from build123d import *

# Parameters (mm, degrees)
SKETCH1_W           = 30
SKETCH1_H           = 10
BOSS_EXTRUDE1_DEPTH = 0.6
SKETCH2_W           = 0.6
SKETCH2_H           = 10
BOSS_EXTRUDE2_DEPTH = 10
FILLET1_R           = 0.5
FILLET2_R           = 3
CUT_EXTRUDE1_REACH  = 2.6
SKETCH3_R           = 2.5


with BuildPart() as part:
    # Sketch1 → Boss-Extrude1 (new body)
    with BuildSketch(Plane(origin=(0, 0, 0), x_dir=(1, 0, 0), z_dir=(0, 1, 0))):
        Rectangle(SKETCH1_W, SKETCH1_H)
    extrude(amount=BOSS_EXTRUDE1_DEPTH)

    # Sketch2 → Boss-Extrude2 (add)
    with BuildSketch(Plane(origin=(0, 0.6, 0), x_dir=(1, 0, 0), z_dir=(0, 1, 0))):
        with Locations((-14.7, 0)):
            Rectangle(SKETCH2_W, SKETCH2_H)
        with Locations((14.7, 0)):
            Rectangle(SKETCH2_W, SKETCH2_H)
    extrude(amount=BOSS_EXTRUDE2_DEPTH)

    # Fillet1
    fillet1_edges = [part.edges().sort_by_distance(p)[0] for p in [
        (-14.4, 0.6, 0),
        (14.4, 0.6, 0),
        (-15, 0, 0),
        (15, 0, 0),
    ]]
    fillet(fillet1_edges, radius=FILLET1_R)

    # Fillet2
    fillet2_edges = [part.edges().sort_by_distance(p)[0] for p in [
        (-14.7, 10.6, 5),
        (-14.7, 10.6, -5),
        (14.7, 10.6, -5),
        (14.7, 10.6, 5),
    ]]
    fillet(fillet2_edges, radius=FILLET2_R)

    # Sketch3 → Cut-Extrude1 (cut, up to next)
    with BuildSketch(Plane(origin=(0, 0.6, 0), x_dir=(1, 0, 0), z_dir=(0, 1, 0)), mode=Mode.PRIVATE) as cut_extrude1_sk1:
        Circle(SKETCH3_R)
    cut_extrude1_tool1 = extrude(cut_extrude1_sk1.sketch, amount=-CUT_EXTRUDE1_REACH, mode=Mode.PRIVATE) & part.part
    add(cut_extrude1_tool1.solids().sort_by_distance((0, 0.6, 0))[0], mode=Mode.SUBTRACT)


solid = part.part
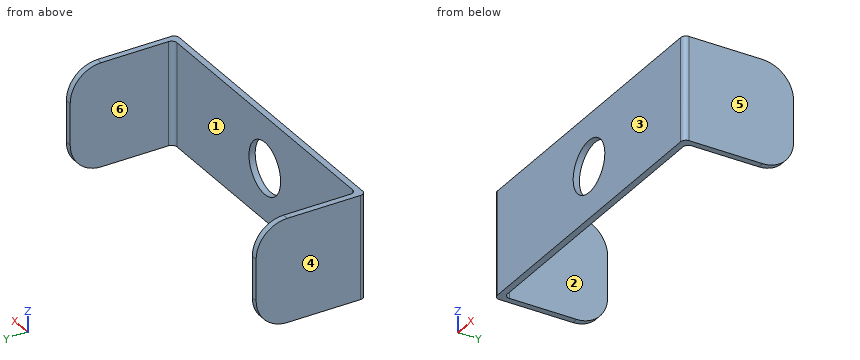
CAD build for the part. Positions are in the model's coordinates, mm. Face numbers are marked on the shaded views. A direction names the side the tool comes from. Give positions to 0.01 mm unless a question says otherwise; leave off trailing zeros. Write each loop counter-clockwise with the first axis right and the second up, starting at its lowest first coordinate (ties: lowest second). Pieces come first, ordered by that corner, then holes. Notation, with made-up numbers: (46.5, -14.5) - (60.5, -14.5) arc R13 cw to (60.5, -10.5) - close; hole circle Ø1 at (14.5, 34). An arc over 180 degrees is marked (long way). Answer as CSV lines item,"result".
Q1. Band-saw the part on B-B (z = 0). Give the cut face in (x, y), and give its area (3 significant figures).
Result set:
outline,"(-15, 0.5) arc R0.5 ccw to (-14.5, 0) - (-2.5, 0) - (-2.5, 0.6) - (-13.9, 0.6) arc R0.5 cw to (-14.4, 1.1) - (-14.4, 10.6) - (-15, 10.6) - close; (2.5, 0) - (14.5, 0) arc R0.5 ccw to (15, 0.5) - (15, 10.6) - (14.4, 10.6) - (14.4, 1.1) arc R0.5 cw to (13.9, 0.6) - (2.5, 0.6) - close"
area,"27.0 mm²"
Q2. Pull direction X, two halves, no side cores. Call the marked faces 1, 2, 3 and 4: released by +X, released by -X, zero draft, split by the parting line, or undercut.
Result set:
face 1,"undercut"
face 2,"undercut"
face 3,"zero draft"
face 4,"released by -X"
Q3. Drill centre lines: line 1 (X direction, y = 9.75, z = 4); line 2 (X direction, y = 0.5, z = 0); line 3 (Z direction, x = 0, y = 0.2). Where is each one in solid material? Low to high. Write a range as from..to.
Result set:
line 1,"-15..-14.4, 14.4..15"
line 2,"-15..-2.5, 2.5..15"
line 3,"-5..-2.5, 2.5..5"
Q4. 3-axis set-ups, long thin cutter, end or side, ignore diameter. For the marked faces 5 and 6: which of +Z, -Z, +X, -X, +Y, -Y reach the whole face in a straight line?
Result set:
face 5,"+Z, -Z, +X, +Y, -Y"
face 6,"+Z, -Z, +Y"
Q5. Band-saw the part on D-D (z = 4). Give the cut face in (x, y), and give its area (3 significant figures).
Result set:
outline,"(-15, 0.5) arc R0.5 ccw to (-14.5, 0) - (14.5, 0) arc R0.5 ccw to (15, 0.5) - (15, 9.84) - (14.4, 9.84) - (14.4, 1.1) arc R0.5 cw to (13.9, 0.6) - (-13.9, 0.6) arc R0.5 cw to (-14.4, 1.1) - (-14.4, 9.84) - (-15, 9.84) - close"
area,"29.1 mm²"
Q6. Band-saw the part on A-A (y = 6.75). Give the cut face in (x, z).
Result set:
outline,"(-15, -5) - (-14.4, -5) - (-14.4, 5) - (-15, 5) - close; (14.4, -5) - (15, -5) - (15, 5) - (14.4, 5) - close"
Q7. Band-saw the part on C-C (x = 0). Give the cut face in (y, z), and give its area (3 significant figures).
Result set:
outline,"(0, -5) - (0.6, -5) - (0.6, -2.5) - (0, -2.5) - close; (0, 2.5) - (0.6, 2.5) - (0.6, 5) - (0, 5) - close"
area,"3.00 mm²"
